Design review of the part built by this model. Coordinates are the model's own, in mm. A direction names the side the tool comes from. Coordinates: 2 decimals unless noted, no trailing zeros. Loops run counter-clockwise (first coordinate to the right, second up) from the corner with the lowest first, then second, coordinate; pieces in that order, holes last. Notation, with made-up numbers: (-17, -23.75) -> (0, -23.75) arc R20 cw to (0, 15.25) -> close; hole circle Ø5 at (39, -32.75). An arc over 180 degrees is marked (long way). One line per item, written item: value. Start each with the question number.
1. Add section D-D on z = 3.65. Write out the cut boundary in (x, y).
2. Add section B-B on x = 0. Write out the cut boundary in (y, z).
3. Draft analysis for pull direction Y (two halves, no side actions). For faces 4 (the flat face through (0, -8.5, 1)), 5 (the flat face through (0, 8, 2)), 6 (the flat face through (-9, -2, 1)), state which applies: pulls with the +Y half, pulls with the -Y half, needs draft (parallel to the pull), parting line crosses it, or undercut.
4. For probe 1 along X at (y, z) = (-1, 2); probe 2 along Y at (x, z) = (8, 1.8); probe 3 along Z at (x, y) = (-4, -2), list the stretches that pass through material, from the lowest coordinate up.
5. Add section C-C on y = -4. Write out the cut boundary in (x, z), plus the area to 3 significant figures.
6. Add section A-A on z = 2.7. Write out the cut boundary in (x, y), plus the area to 3 significant figures.
7. Insertion check: pin 1 (1.5 mm diameter, centred on x = 0.5, y = 3, fed in from +Z). The pin has a flat end and moves straight along its axis. Give the tip position at first contact, or say it passes through.
8. Machinability: for faces 1 (the flat face through (7.76, -0.02, 3.63)), 2 (the flat face through (-9, 2, 1)), 3 (the flat face through (9, -2, 1)), which of the approach directions +Z, -Z, +X, -X, +Y, -Y give a long, thin tool a straight path to every point of the face, cutting with its end or side? Answer none if there is none.
```python
from build123d import *

# Parameters (mm, degrees)
F1_DEPTH  = 1
F2_DEPTH  = 2
F0_W      = 1
F0_H      = 3
F3_DEPTH  = 4
F4_W      = 3
F4_H      = 1.0236278605
F5_DEPTH  = 1.5
F7_DEPTH  = 3
F9_DEPTH  = 2
F10_W     = 8.5
F10_H     = 15
F11_DEPTH = 2


# Not quite as in the source:
# - a feature names something its author has since deleted; it is built from what else it names


with BuildPart() as f1:
    # F0 (on Top) → F1 (new body)
    with BuildSketch(Plane.XY):
        Polygon((-8.5, 7.5), (-8.5, 2), (-8.5, 1.5), (-8.5, -1.5), (-8.5, -2), (-8.5, -7.5), (8.5, -7.5), (8.5, 7.5), align=None)
    extrude(amount=F1_DEPTH)

    # F0 (on Top) → F2 (join)
    with BuildSketch(Plane.XY):
        Polygon((9.5, 8.5), (-9.5, 8.5), (-9.5, 2), (-8.5, 2), (-8.5, 7.5), (8.5, 7.5), (8.5, -7.5), (-8.5, -7.5), (-8.5, -2), (-9.5, -2), (-9.5, -8.5), (9.5, -8.5), align=None)
    extrude(amount=F2_DEPTH)

    # F0 (on Top) → F3 (join)
    with BuildSketch(Plane.XY):
        with Locations((-9, 0)):
            Rectangle(F0_W, F0_H)
    extrude(amount=F3_DEPTH)

    # F4 (on face) → F5 (join)
    with BuildSketch(Plane.YZ.offset(-8.5)):
        with Locations((0, 3.4881860698)):
            Rectangle(F4_W, F4_H)
    extrude(amount=F5_DEPTH)

    # F6 (on face) → F7 (cut)
    with BuildSketch(Plane.XZ.offset(1.5)):
        Polygon((-8.5056265816, 4), (-7, 3.2529253513), (-7, 4), align=None)
    extrude(amount=-F7_DEPTH, mode=Mode.SUBTRACT)

    # F8 (on face) → F9 (cut)
    with BuildSketch(Plane.XY.offset(2)):
        Polygon((9.5, 8.5), (0, 8.5), (0, 7.5), (8.5, 7.5), (8.5, -7.5), (0, -7.5), (0, -8.5), (9.5, -8.5), align=None)
    extrude(amount=-F9_DEPTH, mode=Mode.SUBTRACT)

    # F10 (on face) → F11 (cut)
    with BuildSketch(Plane.XY.offset(1)):
        with Locations((4.25, 0)):
            Rectangle(F10_W, F10_H)
    extrude(amount=-F11_DEPTH, mode=Mode.SUBTRACT)

    # F12: F1 across plane


with BuildPart() as f1_1:
    add(f1.part)
    add(f1.part.mirror(Plane.YZ))


solid = f1_1.part
```
Worked answers:
1. outline: (-9.5, -1.5) -> (-7.8, -1.5) -> (-7.8, 1.5) -> (-9.5, 1.5) -> close; (7.8, -1.5) -> (9.5, -1.5) -> (9.5, 1.5) -> (7.8, 1.5) -> close
2. outline: (-8.5, 0) -> (8.5, 0) -> (8.5, 2) -> (7.5, 2) -> (7.5, 1) -> (-7.5, 1) -> (-7.5, 2) -> (-8.5, 2) -> close
3. face 4: pulls with the -Y half
3. face 5: needs draft
3. face 6: undercut
4. probe 1: x = -9.5 to -8.5, 8.5 to 9.5
4. probe 2: y = -8.5 to -7.5, 7.5 to 8.5
4. probe 3: z = 0 to 1
5. outline: (-9.5, 0) -> (9.5, 0) -> (9.5, 2) -> (8.5, 2) -> (8.5, 1) -> (-8.5, 1) -> (-8.5, 2) -> (-9.5, 2) -> close
5. area: 21.0 mm²
6. outline: (-9.5, -1.5) -> (-8.5, -1.5) -> (-8.5, 1.5) -> (-9.5, 1.5) -> close; (8.5, -1.5) -> (9.5, -1.5) -> (9.5, 1.5) -> (8.5, 1.5) -> close
6. area: 6.00 mm²
7. pin 1: stops at z = 1
8. face 1: +Z, +Y, -Y
8. face 2: +Z, -Z, -X
8. face 3: +Z, -Z, +X
